from build123d import *

# Parameters (mm, degrees)
SKETCH_1_R          = 40
EXTRUDE_1_DEPTH     = 10
FILLET_1_R          = 8
SKETCH_2_R          = 4
CUT_EXTRUDE_1_DEPTH = 10


with BuildPart() as part:
    # 草图1 → 凸台-拉伸1 (new body, symmetric)
    with BuildSketch(Plane(origin=(0, 0, 0), x_dir=(1, 0, 0), z_dir=(0, 1, 0))):
        Circle(SKETCH_1_R)
    extrude(amount=EXTRUDE_1_DEPTH, both=True)

    # 圆角1
    fillet_1_edges = [part.edges().sort_by_distance(p)[0] for p in [
        (-40, -10, 0),
        (-40, 10, 0),
    ]]
    fillet(fillet_1_edges, radius=FILLET_1_R)

    # 草图2 → 切除-拉伸1 (cut, symmetric)
    with BuildSketch(Plane(origin=(0, 0, 0), x_dir=(1, 0, 0), z_dir=(0, 1, 0))):
        Circle(SKETCH_2_R)
    extrude(amount=CUT_EXTRUDE_1_DEPTH, both=True, mode=Mode.SUBTRACT)


solid = part.part
Geometry check sheet. Reference: the model listing, model coordinates, mm. Round coordinates to 2 decimals unless told otherwise and drop trailing zeros. Write each loop counter-clockwise with the first axis right and the second up, starting at its lowest first coordinate (ties: lowest second). Pieces come first, ordered by that corner, then holes.
Item 1: Section check C-C (y = 3). Record the boundary of the cut face in (x, z), plus the area to 3 significant figures.
Determined:
outline: circle Ø79.87 at (0, 0); hole circle Ø8 at (0, 0)
area: 4,960 mm2
Item 2: Section check B-B (z = 0). Record the boundary of the cut face in (x, y).
Determined:
outline: (-40, -2) arc R8 ccw to (-32, -10) - (-4, -10) - (-4, 10) - (-32, 10) arc R8 ccw to (-40, 2) - close; (4, -10) - (32, -10) arc R8 ccw to (40, -2) - (40, 2) arc R8 ccw to (32, 10) - (4, 10) - close
Item 3: Section check A-A (x = 0). Record the boundary of the cut face in (y, z), plus the area to 3 significant figures.
Determined:
outline: (-10, -32) arc R8 ccw to (-2, -40) - (2, -40) arc R8 ccw to (10, -32) - (10, -4) - (-10, -4) - close; (-10, 4) - (10, 4) - (10, 32) arc R8 ccw to (2, 40) - (-2, 40) arc R8 ccw to (-10, 32) - close
area: 1,390 mm2
Item 4: Mould release check, pull along X, two halves, no side actions. Record for faces 1 (the face through (-0.867, 0.14, 3.905)), 2 (the face through (-8.67, 0.03, 39.05)), 3 (the face through (7, -10, 0)): +X half, -X half, draft (parallel to the pull), parting line (faces both ways), or undercut.
Determined:
face 1: undercut
face 2: parting line
face 3: draft
Item 5: Material ranges on line 1 along X through (y, z) = (0.25, 0); line 2 along Z through (x, y) = (0, 6), recorded low to high.
Determined:
line 1: x = -40 to -4, 4 to 40
line 2: z = -38.93 to -4, 4 to 38.93
Item 6: Section check D-D (y = -4). Record the boundary of the cut face in (x, z), plus the area to 3 significant figures.
Determined:
outline: circle Ø79.49 at (0, 0); hole circle Ø8 at (0, 0)
area: 4,910 mm2
Item 7: Go/stop test with flat-tipped pins: pin 1 Ø7 at (x, z) = (0, 0) entering from -Y; pin 2 Ø10 at (y, z) = (-3.5, 21) entering from -X; pin 3 Ø4 at (y, z) = (6.5, 5.5) entering from -X; pin 4 Ø12 at (x, y) = (29.5, -4) entering from +Z. Record where each tip stops, or that it passes through.
Determined:
pin 1: passes through
pin 2: stops at x = -36.6
pin 3: stops at x = -39.26
pin 4: stops at z = 32.23
